```python
from build123d import *

# Parameters (mm, degrees)
SKETCH1_R           = 12.7
BASE_EXTRUDE_DEPTH  = 304.8
SKETCH2_W           = 9.525
SKETCH2_H           = 38.1
BOSS_EXTRUDE1_DEPTH = 263.525
SKETCH3_R           = 4.7625
CUT_EXTRUDE1_DEPTH  = 404.303117433
CIRPATTERN1_COUNT   = 3
SKETCH4_R           = 4.7625
CUT_EXTRUDE2_DEPTH  = 607.93174528
SKETCH5_R           = 4.7625
CUT_EXTRUDE3_DEPTH  = 542.433342309
CIRPATTERN2_COUNT   = 3
FILLET1_R           = 3.175
FILLET2_R           = 3.175
FILLET3_R           = 3.175
SKETCH13_R          = 25.4
EXTRUDE1_DEPTH      = 12.7
FILLET4_R           = 3.175


with BuildPart() as part:
    # Sketch1 → Base-Extrude (new body)
    with BuildSketch(Plane.XY):
        with Locations(Location((0, 0, 0), (0, 0, 180))):
            Circle(SKETCH1_R)
    extrude(amount=BASE_EXTRUDE_DEPTH)

    # Sketch2 → Boss-Extrude1 (add)
    with BuildSketch(Plane(origin=(0, 0, 0), x_dir=(1, 0, 0), z_dir=(0, 1, 0))):
        with Locations((0, -19.05)):
            Rectangle(SKETCH2_W, SKETCH2_H)
    boss_extrude1 = extrude(amount=-BOSS_EXTRUDE1_DEPTH)

    # Sketch3 → Cut-Extrude1 (cut, through all)
    with BuildSketch(Plane.ZY.offset(4.7625)):
        with Locations((31.75, -257.175)):
            Circle(SKETCH3_R)
    extrude(amount=-CUT_EXTRUDE1_DEPTH, mode=Mode.SUBTRACT)

    # CirPattern1: Boss-Extrude1 ×3 about axis
    cirpattern1_axis = Axis((0, 0, 0), (0, 0, 1))
    for i in range(1, CIRPATTERN1_COUNT):
        add(boss_extrude1.rotate(cirpattern1_axis, i * 360 / CIRPATTERN1_COUNT))

    # Sketch4 → Cut-Extrude2 (cut, through all)
    with BuildSketch(Plane(origin=(-194.392750727, 106.733445647, 225.067730564), x_dir=(0.8660254037844363, -0.5000000000000042, 0), z_dir=(-0.5000000000000041, -0.8660254037844362, 0))):
        with Locations((-35.459216735, -193.317730564)):
            Circle(SKETCH4_R)
    extrude(amount=-CUT_EXTRUDE2_DEPTH, mode=Mode.SUBTRACT)

    # Sketch5 → Cut-Extrude3 (cut, through all)
    with BuildSketch(Plane(origin=(132.010089203, 70.716799223, 223.485963444), x_dir=(0.8660254037844434, 0.499999999999992, 0), z_dir=(0.499999999999992, -0.8660254037844434, 0))):
        with Locations((107.492509583, -191.735963444)):
            Circle(SKETCH5_R)
    extrude(amount=-CUT_EXTRUDE3_DEPTH, mode=Mode.SUBTRACT)

    # Sketch8 → Hole1 (revolve, cut)
    with BuildSketch(Plane(origin=(0, -63.5, 0), x_dir=(0, 1, 0), z_dir=(1, 0, 0))):
        Polygon((0, 0), (0, 8.616645174), (1.130299021, 7.937493125), (1.130299021, 6.3499945), (1.422398768, 6.3499945), (1.422398768, 0.002539998), (1.422398768, 0), align=None)
    hole1 = revolve(axis=Axis((0, -63.5, 0), (0, 0, 1)), mode=Mode.SUBTRACT)

    # Sketch10 → Hole2 (revolve, cut)
    with BuildSketch(Plane(origin=(0, -139.7, 0), x_dir=(0, 1, 0), z_dir=(1, 0, 0))):
        Polygon((0, 0), (0, 8.616645174), (1.130299021, 7.937493125), (1.130299021, 6.3499945), (1.422398768, 6.3499945), (1.422398768, 0.002539998), (1.422398768, 0), align=None)
    hole2 = revolve(axis=Axis((0, -139.7, 0), (0, 0, 1)), mode=Mode.SUBTRACT)

    # Sketch12 → Hole3 (revolve, cut)
    with BuildSketch(Plane(origin=(0, -215.9, 0), x_dir=(0, 1, 0), z_dir=(1, 0, 0))):
        Polygon((0, 0), (0, 8.616645174), (1.130299021, 7.937493125), (1.130299021, 6.3499945), (1.422398768, 6.3499945), (1.422398768, 0.002539998), (1.422398768, 0), align=None)
    hole3 = revolve(axis=Axis((0, -215.9, 0), (0, 0, 1)), mode=Mode.SUBTRACT)

    # CirPattern2: Hole1, Hole2, Hole3 ×3 about axis
    cirpattern2_axis = Axis((0, 0, 0), (0, 0, 1))
    add([hole1.rotate(cirpattern2_axis, i * 360 / CIRPATTERN2_COUNT) for i in range(1, CIRPATTERN2_COUNT)], mode=Mode.SUBTRACT)
    add([hole2.rotate(cirpattern2_axis, i * 360 / CIRPATTERN2_COUNT) for i in range(1, CIRPATTERN2_COUNT)], mode=Mode.SUBTRACT)
    add([hole3.rotate(cirpattern2_axis, i * 360 / CIRPATTERN2_COUNT) for i in range(1, CIRPATTERN2_COUNT)], mode=Mode.SUBTRACT)

    # Fillet1
    fillet1_edges = [part.edges().sort_by_distance(p)[0] for p in [
        (-12.577153359, 1.762161564, 19.05),
        (-4.7625, -11.773215098, 19.05),
    ]]
    fillet(fillet1_edges, radius=FILLET1_R - 0.0001)  # a hair under: the kernel refuses the full size

    # Fillet2
    fillet2_edges = [part.edges().sort_by_distance(p)[0] for p in [
        (7.814653359, 10.011053535, 19.05),
        (-7.814653359, 10.011053535, 19.05),
    ]]
    fillet(fillet2_edges, radius=FILLET2_R)

    # Fillet3
    fillet3_edges = [part.edges().sort_by_distance(p)[0] for p in [
        (12.577153359, 1.762161564, 19.05),
        (4.7625, -11.773215098, 19.05),
    ]]
    fillet(fillet3_edges, radius=FILLET3_R)

    # Sketch13 → Extrude1 (add)
    with BuildSketch(Plane.XY.offset(304.8)):
        Circle(SKETCH13_R)
    extrude(amount=-EXTRUDE1_DEPTH)

    # Fillet4
    fillet4_edges = [part.edges().sort_by_distance(p)[0] for p in [
        (-25.4, 0, 304.8),
    ]]
    fillet(fillet4_edges, radius=FILLET4_R)


solid = part.part
```
Work out the finished part from the listing and answer in its coordinate system (mm). A direction names the side the tool comes from. Give positions to 0.01 mm unless a question says otherwise; leave off trailing zeros. Write each loop counter-clockwise with the first axis right and the second up, starting at its lowest first coordinate (ties: lowest second). Pieces come first, ordered by that corner, then holes. Notation, with made-up numbers: (42, 5) - (78, 5) arc R29 cw to (78, 44) - close; hole circle Ø5 at (-11.5, 54.25). An arc over 180 degrees is marked (long way). Use one line per item in the form item = value.
1. Each of these flat-tipped pins is pushed along its axis until it touches: pin 1 Ø1 at (x, z) = (8, 59.5) entering from +Y; pin 2 Ø1.8 at (x, y) = (0, -215.9) entering from +Z; pin 3 Ø2.5 at (x, y) = (0, -139.7) entering from -Z; pin 4 Ø3 at (x, y) = (187.5, 108.5) entering from -Z. Where does it stop, or does it pass through?
Filled in:
pin_1 = 10.25
pin_2 = 38.1
pin_3 = 6.35
pin_4 = 0
2. A cutting plane is placed at A-A (y = 49). Write down the section's boundary in (x, z).
Filled in:
outline = (-94.4, 0) - (-75.35, 0) - (-75.35, 38.1) - (-94.4, 38.1) - close; (75.35, 0) - (94.4, 0) - (94.4, 38.1) - (75.35, 38.1) - close
3. For faces 5 (the face through (-12.114, -3.815, 144.005)), 6 (the face through (0, 0, 304.8)), determine the directions among +Z, -Z, +X, -X, +Y, -Y from which every point of the face is accessible in a straight line to the end or side of a thin tool.
Filled in:
face_5 = none
face_6 = +Z, +X, -X, +Y, -Y
4. A cutting plane is placed at C-C (y = -39.5). Write down the section's boundary in (x, z).
Filled in:
outline = (-4.76, 0) - (4.76, 0) - (4.76, 38.1) - (-4.76, 38.1) - close
5. A cutting plane is placed at B-B (z = 205.5). Write down the section's boundary in (x, y), and give its area (3 significant figures).
Filled in:
outline = circle Ø25.4 at (0, 0)
area = 507 mm^2
6. Determine the mould class of faces 1 (the face through (117, 68, 38.1)), 2 (the face through (120.93, 64.32, 19.32)), 3 (the face through (116.17, 72.57, 19.32)), 4 (the face through (-218.82, 126.26, 33.18)) for opening direction X: released by +X, released by -X, zero draft, split by the parting line, or undercut.
Filled in:
face_1 = zero draft
face_2 = released by +X
face_3 = undercut
face_4 = undercut
7. Consider L1, parallel to Y at x = 0, z = 7.35 (3 decimals); L2, parallel to Y at x = 0, z = 3 (3 decimals); L3, parallel to X at y = 69, z = 5. Determine where each line is inside the solid, lowest interval first.
Filled in:
L1 = -263.525 to -217.03, -214.77 to -140.83, -138.57 to -64.63, -62.37 to 12.7
L2 = -263.525 to -217.322, -214.478 to -141.122, -138.278 to -64.922, -62.078 to 12.7
L3 = -129.04 to -122.12, -119.84 to -109.99, 109.99 to 119.84, 122.12 to 129.04
8. A cutting plane is placed at D-D (x = -197). Write down the section's boundary in (y, z).
Filled in:
outline = (108.24, 0) - (119.24, 0) - (119.24, 38.1) - (108.24, 38.1) - close
